```python
from build123d import *

# Parameters (mm, degrees)
F1_DEPTH = 3.175
F2_DEPTH = 25.4
F3_D     = 7.62


with BuildPart() as f1:
    # F0 (on Top) → F1 (new body)
    with BuildSketch(Plane.XY):
        with BuildLine():
            Line((-5.1198361907, 0), (0, 0))
            Line((0, 0), (0, 14.0471234521))
            ThreePointArc((0, 14.0471234521), (-4.826, 18.8731234521), (0, 23.6991234521))
            Line((0, 23.6991234521), (0, 38.1))
            Line((0, 38.1), (0, 40.3563641012))
            Line((0, 40.3563641012), (9.1353934258, 42.9664775729))
            Line((9.1353934258, 42.9664775729), (0, 42.9664775729))
            ThreePointArc((0, 42.9664775729), (-3.4411192923, 41.5411192923), (-4.8664775729, 38.1))
            Line((-4.8664775729, 38.1), (-5.1198361907, 18.8731234521))
            Line((-5.1198361907, 18.8731234521), (-5.1198361907, 0))
        make_face()
        with BuildLine():
            Line((0, 38.1), (0, 23.6991234521))
            ThreePointArc((0, 23.6991234521), (3.412497326, 22.2856207781), (4.826, 18.8731234521))
            Line((4.826, 18.8731234521), (4.826, 38.1))
            Line((4.826, 38.1), (0, 38.1))
        make_face()
        with BuildLine():
            Line((0, 19.05), (0, 14.0471234521))
            ThreePointArc((0, 14.0471234521), (3.412497326, 15.4606261261), (4.826, 18.8731234521))
            ThreePointArc((4.826, 18.8731234521), (3.412497326, 22.2856207781), (0, 23.6991234521))
            Line((0, 23.6991234521), (0, 19.05))
        make_face()
        with BuildLine():
            ThreePointArc((0, 23.6991234521), (-4.826, 18.8731234521), (0, 14.0471234521))
            Line((0, 14.0471234521), (0, 19.05))
            Line((0, 19.05), (0, 23.6991234521))
        make_face()
        with BuildLine():
            Line((0, 14.0471234521), (0, 0))
            Line((0, 0), (4.826, 0))
            Line((4.826, 0), (4.826, 4.826))
            Line((4.826, 4.826), (4.826, 18.8731234521))
            ThreePointArc((4.826, 18.8731234521), (3.412497326, 15.4606261261), (0, 14.0471234521))
        make_face()
    extrude(amount=F1_DEPTH)

    # F0 (on Top) + F1_face (on face) → F2 (cut)
    with BuildSketch(Plane.XY):
        with BuildLine():
            Line((-5.1198361907, 0), (0, 0))
            Line((0, 0), (0, 14.0471234521))
            ThreePointArc((0, 14.0471234521), (-4.826, 18.8731234521), (0, 23.6991234521))
            Line((0, 23.6991234521), (0, 38.1))
            Line((0, 38.1), (0, 40.3563641012))
            Line((0, 40.3563641012), (9.1353934258, 42.9664775729))
            Line((9.1353934258, 42.9664775729), (0, 42.9664775729))
            ThreePointArc((0, 42.9664775729), (-3.4411192923, 41.5411192923), (-4.8664775729, 38.1))
            Line((-4.8664775729, 38.1), (-5.1198361907, 18.8731234521))
            Line((-5.1198361907, 18.8731234521), (-5.1198361907, 0))
        make_face()
        with BuildLine():
            Line((0, 14.0471234521), (0, 0))
            Line((0, 0), (4.826, 0))
            Line((4.826, 0), (4.826, 4.826))
            Line((4.826, 4.826), (4.826, 18.8731234521))
            ThreePointArc((4.826, 18.8731234521), (3.412497326, 15.4606261261), (0, 14.0471234521))
        make_face()
        with BuildLine():
            Line((0, 19.05), (0, 14.0471234521))
            ThreePointArc((0, 14.0471234521), (3.412497326, 15.4606261261), (4.826, 18.8731234521))
            ThreePointArc((4.826, 18.8731234521), (3.412497326, 22.2856207781), (0, 23.6991234521))
            Line((0, 23.6991234521), (0, 19.05))
        make_face()
        with BuildLine():
            Line((0, 38.1), (0, 23.6991234521))
            ThreePointArc((0, 23.6991234521), (3.412497326, 22.2856207781), (4.826, 18.8731234521))
            Line((4.826, 18.8731234521), (4.826, 38.1))
            Line((4.826, 38.1), (0, 38.1))
        make_face()
    with BuildSketch(Plane(origin=(-0.1118375102, 20.6143518091, 0), x_dir=(1, 0, 0), z_dir=(0, 0, -1))):
        with BuildLine():
            Line((0.1118375102, -17.4856481909), (4.9378375102, -17.4856481909))
            Line((4.9378375102, -17.4856481909), (4.9378375102, 20.6143518091))
            Line((4.9378375102, 20.6143518091), (-5.0079986805, 20.6143518091))
            Line((-5.0079986805, 20.6143518091), (-5.0079986805, 1.741228357))
            Line((-5.0079986805, 1.741228357), (-4.7546400627, -17.4856481909))
            ThreePointArc((-4.7546400627, -17.4856481909), (-3.3292817821, -20.9267674832), (0.1118375102, -22.3521257638))
            Line((0.1118375102, -22.3521257638), (9.247230936, -22.3521257638))
            Line((9.247230936, -22.3521257638), (0.1118375102, -19.7420122921))
            Line((0.1118375102, -19.7420122921), (0.1118375102, -17.4856481909))
        make_face()
    extrude(amount=-F2_DEPTH, dir=(0, 0, 1), mode=Mode.SUBTRACT)

    # F3 (through all)
    with Locations(Plane(origin=(0, 0, 0), x_dir=(1, 0, 0), z_dir=(0, 0, -1))):
        with Locations((0, -19.05)):
            Hole(F3_D / 2)


solid = f1.part
```
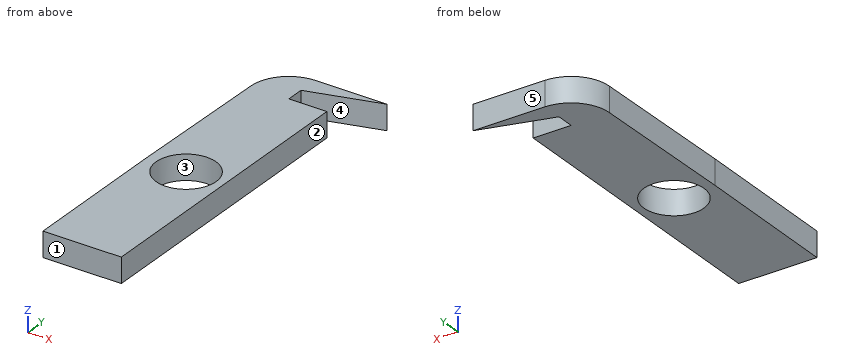
For this review, take the finished solid that the model builds, in its own axes (mm). Face numbers are marked on the shaded views. A direction names the side the tool comes from. Round coordinates to 2 decimals unless told otherwise and drop trailing zeros. Write each loop counter-clockwise with the first axis right and the second up, starting at its lowest first coordinate (ties: lowest second). Pieces come first, ordered by that corner, then holes. Notation, with made-up numbers: (61.5, 50.5) - (117.5, 50.5) arc R15 ccw to (117.5, 63.5) - close; hole circle Ø2 at (88, -21). An arc over 180 degrees is marked (long way). Answer as a JSON object with one key per item and string values.
1. We need section B-B on x = 2.25. Give the boundary of the cut face in (y, z) (3 decimals).
Response values:
{"outline": "(0, 0) - (15.975, 0) - (15.975, 3.175) - (0, 3.175) - close; (22.125, 0) - (38.1, 0) - (38.1, 3.175) - (22.125, 3.175) - close; (40.999, 0) - (42.966, 0) - (42.966, 3.175) - (40.999, 3.175) - close"}
2. Draft analysis for pull direction X (two halves, no side actions). For the marked faces 3, 4 and 5, state which applies: +X half, -X half, draft (parallel to the pull), parting line (faces both ways), or undercut.
Response values:
{"face 3": "undercut", "face 4": "+X half", "face 5": "draft"}
3. We need section A-A on z = 1.15. Give the boundary of the cut face in (x, y), then the cut area to 3 significant figures.
Response values:
{"outline": "(-5.12, 0) - (4.83, 0) - (4.83, 38.1) - (0, 38.1) - (0, 40.36) - (9.14, 42.97) - (0, 42.97) arc R4.87 ccw to (-4.87, 38.1) - (-5.12, 18.87) - close; hole circle Ø7.62 at (0, 19.05)", "area": "361 mm2"}
4. For pin 1 Ø1.6 at (y, z) = (27.5, 1.5) entering from +X; pin 2 Ø1 at (y, z) = (25.5, 0.5) entering from -X, all flat-tipped, find the tip position at first contact; note any pin that passes through.
Response values:
{"pin 1": "stops at x = 4.83", "pin 2": "stops at x = -5.04"}
5. To check wall thickness, follow line 1 along X through (y, z) = (19.05, 2.1); line 2 along Y through (x, z) = (2, 1.1); line 3 along Y through (x, z) = (-3, 1.5). State the ranges of each line that lie inside material, in increasing order.
Response values:
{"line 1": "x = -5.12 to -3.81, 3.81 to 4.83", "line 2": "y = 0 to 15.81, 22.29 to 38.1, 40.93 to 42.97", "line 3": "y = 0 to 16.7, 21.4 to 41.93"}
6. Tool access review of the marked faces 1 and 2: name each direction out of +Z, -Z, +X, -X, +Y, -Y from which nothing blocks a thin tool from reaching the whole face with its end or side.
Response values:
{"face 1": "+Z, -Z, +X, -X, -Y", "face 2": "+Z, -Z, +X, -Y"}
7. We need section C-C on x = -2. Give the boundary of the cut face in (y, z) (1 decimal).
Response values:
{"outline": "(0, 0) - (15.8, 0) - (15.8, 3.2) - (0, 3.2) - close; (22.3, 0) - (42.5, 0) - (42.5, 3.2) - (22.3, 3.2) - close"}
8. We need section D-D on y = 18. Give the boundary of the cut face in (x, z) (3 decimals).
Response values:
{"outline": "(-5.12, 0) - (-3.662, 0) - (-3.662, 3.175) - (-5.12, 3.175) - close; (3.662, 0) - (4.826, 0) - (4.826, 3.175) - (3.662, 3.175) - close"}
